Design review of the part shown in the three views and the two pictorial views. Dimensions are in mm from the part's minimum x, y and z. Coordinates: 2 decimals unless noted, no trailing zeros. Write each loop counter-clockwise with the first axis right and the second up, starting at its lowest first coordinate (ties: lowest second). Pieces come first, ordered by that corner, then holes. Notation, with made-up numbers: M 48,-29 L 63,-29 A23 cw 63,6 Z; hole C 48,49 d3. An arc over 180 degrees is marked long. Answer as a JSON object with one key per item and string values.
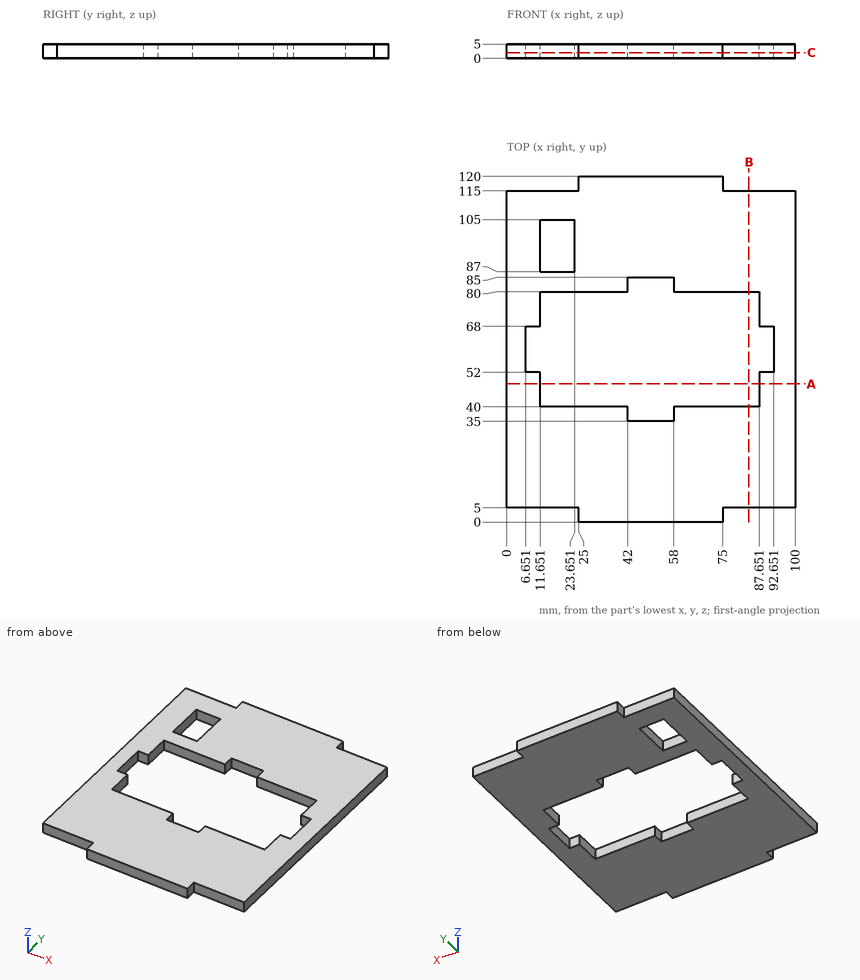
(1) Wall thickness on line 1 along Y through (x, z) = (20.5, 3.45); line 2 along Y through (x, z) = (54.5, 2.6); line 3 along X through (y, z) = (64, 3.75): over which ranges is each line inside the solid? List them lowest first. Write a range as from..to.
Results list:
{"line 1": "5..40, 80..87, 105..115", "line 2": "0..35, 85..120", "line 3": "0..6.65, 92.65..100"}
(2) Add section C-C on z = 2.05. Count the separate pieces of the cut face and the enclosed holes in it, and give its area (3 significant figures).
Results list:
{"separate pieces": "1", "enclosed holes": "2", "area": "7,920 mm²"}
(3) Add section A-A on y = 48. Give the boundary of the cut face in (x, z).
Results list:
{"outline": "M 0,0 L 11.65,0 L 11.65,5 L 0,5 Z; M 87.65,0 L 100,0 L 100,5 L 87.65,5 Z"}
(4) For pin 1 Ø2.5 at (x, z) = (12.5, 2.5) entering from +Y; pin 2 Ø1.5 at (x, z) = (81.5, 1.5) entering from -Y; pin 3 Ø1.5 at (y, z) = (118, 1.5) entering from +X, all flat-tipped, find the tip position at first contact; note any pin that passes through.
Results list:
{"pin 1": "y = 115", "pin 2": "y = 5", "pin 3": "x = 75"}
(5) Add section B-B on x = 84. Give the boundary of the cut face in (y, z), and give its area (3 significant figures).
Results list:
{"outline": "M 5,0 L 40,0 L 40,5 L 5,5 Z; M 80,0 L 115,0 L 115,5 L 80,5 Z", "area": "350 mm²"}
